Check sheet for the modelled part. Datum: model origin and axes. Units: mm. A direction names the side the tool comes from. Round coordinates to 2 decimals unless told otherwise and drop trailing zeros. Loops run counter-clockwise (first coordinate to the right, second up) from the corner with the lowest first, then second, coordinate; pieces in that order, holes last. Notation, with made-up numbers: (-6, -13) -> (38, -13) arc R26 ccw to (38, 15) -> close; hole circle Ø7 at (78, 61.25). An arc over 180 degrees is marked (long way). Use one line per item in the form item = value. Start each with the question number.
(1) Sectioned sample at B-B (z = 0). Record the cut outline in (x, y).
(2) Sectioned sample at A-A (x = 6.5). Record the cut outline in (y, z), and give its area (3 significant figures).
(3) Draft check along Y on faces 5 (the flat face through (6, 18.2, -2)), 6 (the flat face through (0, 0, 0)), 7 (the cylindrical face through (7.81, 14.46, 1.73)). Enter one of: released by +Y, released by -Y, zero draft, split by the parting line, or undercut.
(4) Sectioned sample at D-D (y = 3.5). Record the cut outline in (x, z), and give its area (3 significant figures).
(5) Go/stop test with flat-tipped pins: pin 1 (1 mm diameter, centred on x = 0.5, y = 4, fed in from +Z); pin 2 (2 mm diameter, centred on y = 11, z = -6, fed in from +X); pin 3 (4 mm diameter, centred on x = -3, y = 17, fed in from -Z). Record where each tip stops, or that it passes through.
(6) Set-up check for faces 1 (the flat face through (-6, 13.7, 2)), 2 (the cylindrical face through (-2.777, 19.087, 6.697)), 3 (the flat face through (0, 20, 0)), 4 (the flat face through (-6, 15.2, 2)): record each of +Z, -Z, +X, -X, +Y, -Y from which the full face is reachable in a straight line by a thin tool's end or side.
(7) Sectioned sample at C-C (x = 0). Record the cut outline in (y, z), and give its area (4 significant figures).
(8) Material ranges on probe 1 along Y at (x, z) = (5.25, 4.5); probe 2 along Y at (x, z) = (-7, 3); probe 3 along Z at (x, y) = (1, 12.25), recorded low to high. Write a range as [from, to].
from build123d import *

# Parameters (mm, degrees)
SKETCH_1_R      = 6
EXTRUDE_1_DEPTH = 18.2
SKETCH_2_R      = 7.25
EXTRUDE_2_DEPTH = 1.8
SKETCH_3_W      = 2
SKETCH_3_H      = 1.5


with BuildPart() as part:
    # 草图1 → 凸台-拉伸1 (new body)
    with BuildSketch(Plane(origin=(0, 0, 0), x_dir=(1, 0, 0), z_dir=(0, 1, 0))):
        with Locations(Location((0, 0, 0), (0, 0, 270))):
            Circle(SKETCH_1_R)
    extrude(amount=EXTRUDE_1_DEPTH)

    # 草图2 → 凸台-拉伸2 (add)
    with BuildSketch(Plane(origin=(0, 18.2, 0), x_dir=(1, 0, 0), z_dir=(0, 1, 0))):
        with Locations(Location((0, 0, 0), (0, 0, 270))):
            Circle(SKETCH_2_R)
    extrude(amount=EXTRUDE_2_DEPTH)

    # 草图3 → 旋转1 (revolve)
    with BuildSketch(Plane(origin=(0, 0, 0), x_dir=(0, 0, -1), z_dir=(1, 0, 0)), mode=Mode.PRIVATE) as revolve_1_sk:
        with Locations((-7, 14.45)):
            Rectangle(SKETCH_3_W, SKETCH_3_H)
    revolve(revolve_1_sk.sketch.rotate(Axis((0, 0, 0), (0, 1, 0)), 180), axis=Axis((0, 0, 0), (0, 1, 0)))


solid = part.part
Checks:
q1.outline = (-8, 13.7) -> (-6, 13.7) -> (-6, 0) -> (6, 0) -> (6, 13.7) -> (8, 13.7) -> (8, 15.2) -> (6, 15.2) -> (6, 18.2) -> (7.25, 18.2) -> (7.25, 20) -> (-7.25, 20) -> (-7.25, 18.2) -> (-6, 18.2) -> (-6, 15.2) -> (-8, 15.2) -> close
q2.outline = (13.7, -4.66) -> (15.2, -4.66) -> (15.2, 4.66) -> (13.7, 4.66) -> close; (18.2, -3.21) -> (20, -3.21) -> (20, 3.21) -> (18.2, 3.21) -> close
q2.area = 25.6 mm2
q3.face_5 = undercut
q3.face_6 = released by -Y
q3.face_7 = zero draft
q4.outline = circle Ø12 at (0, 0)
q4.area = 113 mm2
q5.pin_1 = 6
q5.pin_2 = 3.32
q5.pin_3 = -7.71
q6.face_1 = -Y
q6.face_2 = +Y
q6.face_3 = +Z, -Z, +X, -X, +Y
q6.face_4 = none
q7.outline = (0, -6) -> (13.7, -6) -> (13.7, -8) -> (15.2, -8) -> (15.2, -6) -> (18.2, -6) -> (18.2, -7.25) -> (20, -7.25) -> (20, 7.25) -> (18.2, 7.25) -> (18.2, 6) -> (15.2, 6) -> (15.2, 8) -> (13.7, 8) -> (13.7, 6) -> (0, 6) -> close
q7.area = 250.5 mm2
q8.probe_1 = [13.7, 15.2], [18.2, 20]
q8.probe_2 = [13.7, 15.2]
q8.probe_3 = [-5.92, 5.92]
